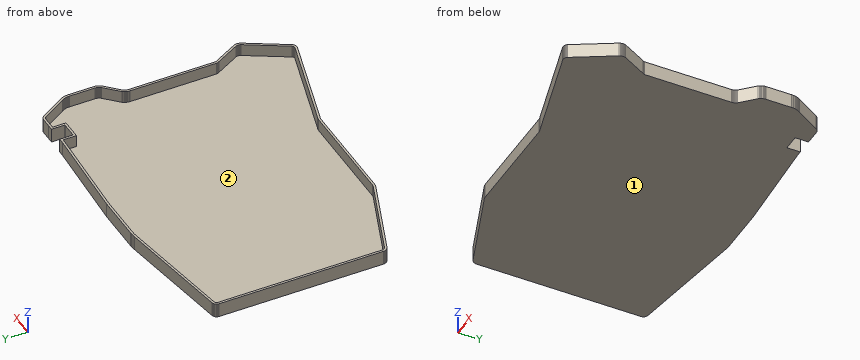
from build123d import *

# Parameters (mm, degrees)
BOSS_EXTRU_1_DEPTH = 6.5
COQUE1_T           = -1


with BuildPart() as part:
    # Esquisse1 → Boss.-Extru.1 (new body)
    with BuildSketch(Plane.XY):
        Polygon((121.817464, 7.492943), (119.344698096, 7.492943), (76.183818096, 9.845583), (55.564779836, 9.845583), (54.552173404, 9.812435234), (53.533209696, 9.726302114), (52.535480793, 9.589824274), (0.457881428, 1.377587451), (0.080923827, 1.263928085), (-0.29188868, 1.068065272), (-0.62076937, 0.805019767), (-0.893764513, 0.484354906), (-1.100960827, 0.11771658), (-1.234846295, -0.281630821), (-1.286572721, -0.669801542), (-1.313614475, -74.551979081), (-1.278040024, -74.923678753), (-1.183440664, -75.310181205), (-1.034124026, -75.679013791), (-0.83321163, -76.022476002), (-0.584894436, -76.333396945), (-0.29436239, -76.605283146), (0.032415912, -76.832524633), (0.369780396, -77.00084256), (36.304970835, -90.526464897), (36.80277452, -90.74345953), (37.387467468, -90.935559968), (37.987559572, -91.072151235), (38.615965116, -91.154417), (85.623172099, -91.154417), (86.041723807, -91.203108273), (86.479101326, -91.284778635), (86.909816867, -91.396315659), (87.386772904, -91.555543407), (131.068933438, -103.89053292), (131.455504757, -103.929660689), (131.837402239, -103.90606587), (132.210442209, -103.820965251), (132.564787964, -103.676607455), (132.89109687, -103.476794608), (133.180788715, -103.226774051), (133.429739598, -102.92886536), (143.750781449, -85.005495121), (143.915060156, -84.629514823), (144.034345378, -84.231627617), (144.104871469, -83.822278759), (144.125612773, -83.407413185), (144.096265486, -82.993066766), (144.017262186, -82.585292428), (143.880179871, -82.160245981), (138.026657959, -71.311045886), (137.876543424, -71.058845944), (137.78546804, -70.860016908), (137.716227615, -70.652585277), (137.681143, -70.491756357), (137.681143, -31.622548821), (137.6990854, -31.232462255), (137.749599164, -30.868463071), (137.833314637, -30.510636851), (137.949524742, -30.162007333), (138.097248212, -29.82551681), (138.275237168, -29.504008987), (138.454865034, -29.240054529), (144.543883236, -23.151036326), (144.845002348, -22.736623208), (145.089736472, -22.322824981), (145.294432727, -21.887826778), (145.457273896, -21.435491716), (145.576812433, -20.969836233), (145.651988542, -20.494996542), (145.681143, -20.030945018), (145.681143, -8.589075407), (145.669842672, -8.050387206), (145.61465745, -7.486457006), (145.516495569, -6.928400528), (145.37593068, -6.379489779), (145.193788673, -5.842940054), (144.971135156, -5.321894978), (144.70927891, -4.819414981), (144.433744876, -4.376954091), (137.970333494, 6.337024694), (137.701988909, 6.669821714), (137.372955521, 6.963781332), (137.000567914, 7.200433726), (136.594704241, 7.373498612), (136.166125996, 7.47838751), (135.767380568, 7.509136644), (131.515559688, 7.492943), (129.017464, 7.492943), (129.017464, 1.492943), (121.817464, 1.492943), align=None)
    extrude(amount=-BOSS_EXTRU_1_DEPTH)

    # Coque1
    coque1_openings = [part.faces().sort_by_distance(p)[0] for p in [
        (72.557857735, -42.2287033, 0),
    ]]
    offset(amount=COQUE1_T, openings=coque1_openings, kind=Kind.INTERSECTION)


solid = part.part
Work out the finished part from the listing and answer in its coordinate system (mm). Face numbers are marked on the shaded views. Coordinates: 2 decimals unless noted, no trailing zeros. Loops run counter-clockwise (first coordinate to the right, second up) from the corner with the lowest first, then second, coordinate; pieces in that order, holes last. Notation, with made-up numbers: (-7.75, -38.5) -> (39.25, -38.5) arc R23 ccw to (39.25, -8.5) -> close; hole circle Ø3 at (-34, 47). An arc over 180 degrees is marked (long way). Write each question's results on one line, items separated by ' | '. Start each with the question number.
1) Consider line 1 along X through (y, z) = (-20, -0.5); line 2 along Y through (x, z) = (75, -2.75); line 3 along X through (y, z) = (-66.5, -3.5). Determine where each line is inside the solid, lowest interval first.
2) Find section B-B on y = -53. Determine the outline of the cut face in (x, z).
3) Find section A-A on x = 74. Determine the outline of the cut face in (y, z).
4) The mould has two halves that part along Y. Classify the marked faces 1 and 2: pulls with the +Y half, pulls with the -Y half, needs draft (parallel to the pull), parting line crosses it, or undercut.
5) Flat-ended cylindrical pins translate along their axes: P1, Ø1.5, axis at x = 122.5, y = -46, coming from the +Z side; P2, Ø2, axis at y = -45.5, z = -2.5, coming from the +X side; P3, Ø1.6, axis at x = 120, z = -1.5, coming from the -Y side. Find the tip coordinate at first contact, or state that the pin passes through.
Response values:
1) line 1: x = -1.29 to -0.29, 144.68 to 145.68 | line 2: y = -91.15 to -90.15, 8.85 to 9.85 | line 3: x = -1.31 to -0.31, 136.68 to 137.68
2) outline: (-1.31, -6.5) -> (137.68, -6.5) -> (137.68, 0) -> (136.68, 0) -> (136.68, -5.5) -> (-0.31, -5.5) -> (-0.31, 0) -> (-1.31, 0) -> close
3) outline: (-91.15, -6.5) -> (9.85, -6.5) -> (9.85, 0) -> (8.85, 0) -> (8.85, -5.5) -> (-90.15, -5.5) -> (-90.15, 0) -> (-91.15, 0) -> close
4) face 1: needs draft | face 2: undercut
5) P1: stops at z = -5.5 | P2: stops at x = 137.68 | P3: stops at y = -100.99
